from build123d import *

# Parameters (mm, degrees)
F1_DEPTH = 15.24
F2_DEPTH = 25.4


with BuildPart() as f1:
    # F0 (on Top) → F1 (new body)
    with BuildSketch(Plane.XY):
        Polygon((-378.244507, 292.142749), (-756.070369, 292.142749), (-756.070369, -228.557251), (-0.418645, -228.577329), (-0.418645, 292.142749), align=None)
        with BuildLine():
            ThreePointArc((-718.259513, 230.902804), (-710.820026, 248.863316), (-692.859513, 256.302804))
            Line((-692.859513, 256.302804), (-441.455363, 256.302804))
            ThreePointArc((-441.455363, 256.302804), (-423.49485, 248.863316), (-416.055363, 230.902804))
            Line((-416.055363, 230.902804), (-416.055363, -167.317306))
            ThreePointArc((-416.055363, -167.317306), (-423.49485, -185.277818), (-441.455363, -192.717306))
            Line((-441.455363, -192.717306), (-692.859513, -192.717306))
            ThreePointArc((-692.859513, -192.717306), (-710.820026, -185.277818), (-718.259513, -167.317306))
            Line((-718.259513, -167.317306), (-718.259513, 230.902804))
        make_face(mode=Mode.SUBTRACT)
        with BuildLine():
            Line((-337.259513, -167.317306), (-337.259513, 230.902804))
            ThreePointArc((-337.259513, 230.902804), (-329.820026, 248.863316), (-311.859513, 256.302804))
            Line((-311.859513, 256.302804), (-60.455363, 256.302804))
            ThreePointArc((-60.455363, 256.302804), (-42.49485, 248.863316), (-35.055363, 230.902804))
            Line((-35.055363, 230.902804), (-35.055363, -167.317306))
            ThreePointArc((-35.055363, -167.317306), (-42.49485, -185.277818), (-60.455363, -192.717306))
            Line((-60.455363, -192.717306), (-311.859513, -192.717306))
            ThreePointArc((-311.859513, -192.717306), (-329.820026, -185.277818), (-337.259513, -167.317306))
        make_face(mode=Mode.SUBTRACT)
        Polygon((-0.418645, 292.142749), (-0.418645, -228.577329), (377.405493, -228.577329), (377.405493, 293.284322), align=None)
        with BuildLine():
            Line((43.740487, -167.317306), (43.740487, 230.902804))
            ThreePointArc((43.740487, 230.902804), (51.179974, 248.863316), (69.140487, 256.302804))
            Line((69.140487, 256.302804), (320.544637, 256.302804))
            ThreePointArc((320.544637, 256.302804), (338.50515, 248.863316), (345.944637, 230.902804))
            Line((345.944637, 230.902804), (345.944637, -167.317306))
            ThreePointArc((345.944637, -167.317306), (338.50515, -185.277818), (320.544637, -192.717306))
            Line((320.544637, -192.717306), (69.140487, -192.717306))
            ThreePointArc((69.140487, -192.717306), (51.179974, -185.277818), (43.740487, -167.317306))
        make_face(mode=Mode.SUBTRACT)
        Polygon((377.405493, 293.284322), (377.405493, -228.577329), (755.229631, -228.577329), (755.229631, 294.425895), align=None)
        with BuildLine():
            Line((424.740487, -167.317306), (424.740487, 230.902804))
            ThreePointArc((424.740487, 230.902804), (432.179974, 248.863316), (450.140487, 256.302804))
            Line((450.140487, 256.302804), (701.544637, 256.302804))
            ThreePointArc((701.544637, 256.302804), (719.50515, 248.863316), (726.944637, 230.902804))
            Line((726.944637, 230.902804), (726.944637, -167.317306))
            ThreePointArc((726.944637, -167.317306), (719.50515, -185.277818), (701.544637, -192.717306))
            Line((701.544637, -192.717306), (450.140487, -192.717306))
            ThreePointArc((450.140487, -192.717306), (432.179974, -185.277818), (424.740487, -167.317306))
        make_face(mode=Mode.SUBTRACT)
    extrude(amount=F1_DEPTH)

    # F0 (on Top) → F2 (join)
    with BuildSketch(Plane.XY):
        with BuildLine():
            Line((-441.455363, 256.302804), (-692.859513, 256.302804))
            ThreePointArc((-692.859513, 256.302804), (-710.820026, 248.863316), (-718.259513, 230.902804))
            Line((-718.259513, 230.902804), (-718.259513, -167.317306))
            ThreePointArc((-718.259513, -167.317306), (-710.820026, -185.277818), (-692.859513, -192.717306))
            Line((-692.859513, -192.717306), (-441.455363, -192.717306))
            ThreePointArc((-441.455363, -192.717306), (-423.49485, -185.277818), (-416.055363, -167.317306))
            Line((-416.055363, -167.317306), (-416.055363, 230.902804))
            ThreePointArc((-416.055363, 230.902804), (-423.49485, 248.863316), (-441.455363, 256.302804))
        make_face()
        with BuildLine():
            ThreePointArc((-311.859513, 256.302804), (-329.820026, 248.863316), (-337.259513, 230.902804))
            Line((-337.259513, 230.902804), (-337.259513, -167.317306))
            ThreePointArc((-337.259513, -167.317306), (-329.820026, -185.277818), (-311.859513, -192.717306))
            Line((-311.859513, -192.717306), (-60.455363, -192.717306))
            ThreePointArc((-60.455363, -192.717306), (-42.49485, -185.277818), (-35.055363, -167.317306))
            Line((-35.055363, -167.317306), (-35.055363, 230.902804))
            ThreePointArc((-35.055363, 230.902804), (-42.49485, 248.863316), (-60.455363, 256.302804))
            Line((-60.455363, 256.302804), (-311.859513, 256.302804))
        make_face()
        with BuildLine():
            ThreePointArc((69.140487, 256.302804), (51.179974, 248.863316), (43.740487, 230.902804))
            Line((43.740487, 230.902804), (43.740487, -167.317306))
            ThreePointArc((43.740487, -167.317306), (51.179974, -185.277818), (69.140487, -192.717306))
            Line((69.140487, -192.717306), (320.544637, -192.717306))
            ThreePointArc((320.544637, -192.717306), (338.50515, -185.277818), (345.944637, -167.317306))
            Line((345.944637, -167.317306), (345.944637, 230.902804))
            ThreePointArc((345.944637, 230.902804), (338.50515, 248.863316), (320.544637, 256.302804))
            Line((320.544637, 256.302804), (69.140487, 256.302804))
        make_face()
        with BuildLine():
            ThreePointArc((450.140487, 256.302804), (432.179974, 248.863316), (424.740487, 230.902804))
            Line((424.740487, 230.902804), (424.740487, -167.317306))
            ThreePointArc((424.740487, -167.317306), (432.179974, -185.277818), (450.140487, -192.717306))
            Line((450.140487, -192.717306), (701.544637, -192.717306))
            ThreePointArc((701.544637, -192.717306), (719.50515, -185.277818), (726.944637, -167.317306))
            Line((726.944637, -167.317306), (726.944637, 230.902804))
            ThreePointArc((726.944637, 230.902804), (719.50515, 248.863316), (701.544637, 256.302804))
            Line((701.544637, 256.302804), (450.140487, 256.302804))
        make_face()
    extrude(amount=F2_DEPTH)


solid = f1.part
Input: part model. Units: mm. Frame: model coordinates. A direction names the side the tool comes from. Give positions to 0.01 mm unless a question says otherwise; leave off trailing zeros. Write each loop counter-clockwise with the first axis right and the second up, starting at its lowest first coordinate (ties: lowest second). Pieces come first, ordered by that corner, then holes.
Q1. Material intervals for probe 1 along X at (y, z) = (-13, 18.75); probe 2 along Y at (x, z) = (126.5, 23.25); probe 3 along Y at (x, z) = (101, 7), sorted ascending.
Q2. Section D-D, the plane x = -219. Output: boundary loops of the cut face in (y, z).
Q3. First-contact query: P1, Ø3, axis at x = -517.5, z = 19.5, coming from the +Y side; P2, Ø1.5, axis at x = -61, z = 20.5, coming from the -Y side; P3, Ø11, axis at y = 60, z = 22, coming from the -X side. Flat tips, straight axial feed; report the tip coordinate or a pass-through.
Q4. Section A-A, the plane z = 21.5. State how many separate pieces and enclosed holes the cut face has, plus the area to 3 significant figures.
Q5. Section C-C, the plane x = 240. Output: boundary loops of the cut face in (y, z), plus the area to 3 significant figures.
Q6. Section B-B, the plane y = 30.5. Output: boundary loops of the cut face in (x, z), plus the area to 3 significant figures.
Q7. Set-up query: faces 4 (the face through (719.31, -185.47, 20.25)), 5 (the face through (-711.016, -185.079, 20.249)), 6 (the face through (51.38, 249.06, 20.25)), 7 (the face through (-11, 37, 15.24)), 8 (the face through (-423.69, -185.47, 20.25)). Return all of +Z, -Z, +X, -X, +Y, -Y with unobstructed straight access to the full face (end or side cutting, diameter ignored); none if empty.
Q8. Pull-direction query (X, two-part tool) for faces 1 (the face through (719.702, 248.665, 20.249)), 2 (the face through (193, 35, 25.4)), 3 (the face through (338.702, 248.665, 20.249)); classes: pulls with the +X half, pulls with the -X half, needs draft (parallel to the pull), parting line crosses it, or undercut.
Filled in:
1. probe 1: x = -718.26 to -416.06, -337.26 to -35.06, 43.74 to 345.94, 424.74 to 726.94
1. probe 2: y = -192.72 to 256.3
1. probe 3: y = -228.58 to 292.45
2. outline: (-228.57, 0) - (292.14, 0) - (292.14, 15.24) - (256.3, 15.24) - (256.3, 25.4) - (-192.72, 25.4) - (-192.72, 15.24) - (-228.57, 15.24) - close
3. P1: stops at y = 256.3
3. P2: stops at y = -192.72
3. P3: stops at x = -718.26
4. separate pieces: 4
4. enclosed holes: 0
4. area: 541,000 mm2
5. outline: (-228.58, 0) - (292.87, 0) - (292.87, 15.24) - (256.3, 15.24) - (256.3, 25.4) - (-192.72, 25.4) - (-192.72, 15.24) - (-228.58, 15.24) - close
5. area: 12,500 mm2
6. outline: (-756.07, 0) - (755.23, 0) - (755.23, 15.24) - (726.94, 15.24) - (726.94, 25.4) - (424.74, 25.4) - (424.74, 15.24) - (345.94, 15.24) - (345.94, 25.4) - (43.74, 25.4) - (43.74, 15.24) - (-35.06, 15.24) - (-35.06, 25.4) - (-337.26, 25.4) - (-337.26, 15.24) - (-416.06, 15.24) - (-416.06, 25.4) - (-718.26, 25.4) - (-718.26, 15.24) - (-756.07, 15.24) - close
6. area: 35,300 mm2
7. face 4: +Z, +X, -Y
7. face 5: +Z, -X, -Y
7. face 6: +Z, +Y
7. face 7: +Z
7. face 8: +Z, -Y
8. face 1: pulls with the +X half
8. face 2: needs draft
8. face 3: undercut
